Build history of the part. All positions in model axes, mm. A direction names the side the tool comes from. Round coordinates to 2 decimals unless told otherwise and drop trailing zeros. Loops run counter-clockwise (first coordinate to the right, second up) from the corner with the lowest first, then second, coordinate; pieces in that order, holes last.
from build123d import *

# Parameters (mm, degrees)
F0_W     = 254
F0_H     = 304.8
F1_DEPTH = 9.525
F2_R     = 9.52499
F3_W     = 19.05
F3_H     = 76.2
F4_DEPTH = 19.051


# Not quite as in the source:
# - a fillet or chamfer is up to 0.001 mm smaller than in the source, because OpenCascade refuses the exact size
# - a feature names something its author has since deleted; it is built from what else it names


with BuildPart() as f1:
    # F0 (on Right) → F1 (new body, symmetric)
    with BuildSketch(Plane.YZ):
        Rectangle(F0_W, F0_H)
    extrude(amount=F1_DEPTH, both=True)

    # F2 (radius 9.525 in the source; OpenCascade refuses exactly that, so slightly less here)
    f2_edges = [f1.edges().sort_by_distance(p)[0] for p in [
        (9.525, -127, 0),
        (-9.525, -127, 0),
    ]]
    fillet(f2_edges, radius=F2_R)

    # F3 (on face) → F4 (cut, through all)
    with BuildSketch(Plane.YZ.offset(9.525)):
        with Locations((117.475, 95.25)):
            Rectangle(F3_W, F3_H)
        with Locations((117.475, 0)):
            Rectangle(F3_W, F3_H)
        with Locations((117.475, -95.25)):
            Rectangle(F3_W, F3_H)
    extrude(amount=-F4_DEPTH, mode=Mode.SUBTRACT)


solid = f1.part
(1) Slice it at B-B on x = -4.25. List the corners of the cut face in (y, z), plus the area to 3 significant figures.
Responses:
outline: (-126, -152.4) - (127, -152.4) - (127, -133.35) - (107.95, -133.35) - (107.95, -57.15) - (127, -57.15) - (127, -38.1) - (107.95, -38.1) - (107.95, 38.1) - (127, 38.1) - (127, 57.15) - (107.95, 57.15) - (107.95, 133.35) - (127, 133.35) - (127, 152.4) - (-126, 152.4) - close
area: 72,800 mm2
(2) Which spindle directions (+Z, -Z, +X, -X, +Y, -Y) get a long thin tool onto all of the face, cutting with end or side? Do faces 1 (the face through (0, 107.95, 95)), 2 (the face through (0, 127, 143)). Say none if no direction does.
Responses:
face 1: +X, -X, +Y
face 2: +Z, -Z, +X, -X, +Y
(3) Probe line 1 (Z direction, x = 8.25, y = 115); line 2 (Y direction, x = -0.25, z = 26.5); line 3 (Y direction, x = -1.25, z = -68). List the from-to ranges inside material, lowest first.
Responses:
line 1: z = -152.4 to -133.35, -57.15 to -38.1, 38.1 to 57.15, 133.35 to 152.4
line 2: y = -127 to 107.95
line 3: y = -126.92 to 107.95
(4) Pull direction Z, two halves, no side cores. Call faces 3 (the face through (0, 107.95, -1)), 4 (the face through (0, -2, -152.4)), 5 (the face through (0, 117, 133.35)), 6 (the face through (0, 127, -143)): +Z half, -Z half, draft (parallel to the pull), parting line (faces both ways), or undercut.
Responses:
face 3: undercut
face 4: -Z half
face 5: undercut
face 6: draft
(5) Pin check, flat tips, straight feed: P1, Ø9.5, axis at x = 2, z = 89, coming from the +Y side; P2, Ø3, axis at x = -6.5, z = -27, coming from the -Y side. Stop position of each tip, or through.
Responses:
P1: stops at y = 107.95
P2: stops at y = -125.58
